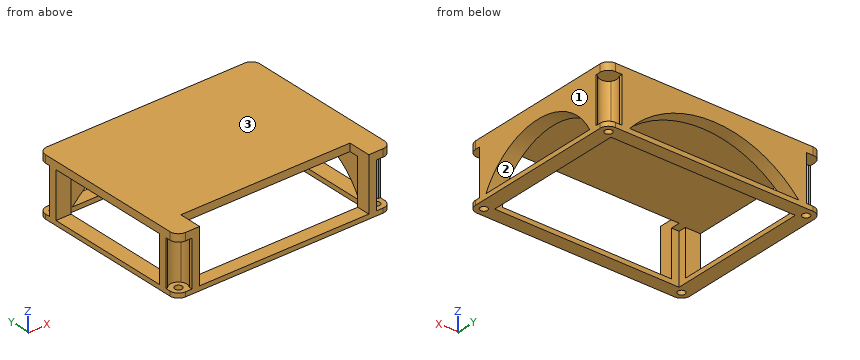
Autodesk Inventor part; units mm, degrees
ref_plane "YZ Plane" through (0, 0, 0) normal (1, 0, 0) x (0, 1, 0)
ref_plane "XZ Plane" through (0, 0, 0) normal (0, 1, 0) x (-1, 0, 0)
ref_plane "XY Plane" through (0, 0, 0) normal (0, 0, 1) x (1, 0, 0)
sketch "Sketch1" plane through (0, 0, 0) normal (0, 0, 1) x (1, 0, 0)
  line L0 (-65, -49.5) -> (65, -49.5) construction
  line L1 (65, -49.5) -> (65, 49.5) construction
  line L2 (65, 49.5) -> (-65, 49.5) construction
  line L3 (-65, 49.5) -> (-65, -49.5) construction
  line L4 (-65, -49.5) -> (65, 49.5) construction
  line L5 (65, -49.5) -> (-65, 49.5) construction
  arc A0 (-65, 55) -> (-70.5, 49.5) centre (-65, 49.5) ccw
  arc A1 (70.5, 49.5) -> (65, 55) centre (65, 49.5) ccw
  arc A2 (65, -55) -> (70.5, -49.5) centre (65, -49.5) ccw
  arc A3 (-70.5, -49.5) -> (-65, -55) centre (-65, -49.5) ccw
  line L6 (-70.5, 49.5) -> (-70.5, -49.5)
  line L7 (-65, -55) -> (65, -55)
  line L8 (70.5, -49.5) -> (70.5, 49.5)
  line L9 (65, 55) -> (-65, 55)
  line L10 (-60.6244, -46.1678) -> (-60.6244, 46.1678)
  line L11 (-60.6244, 46.1678) -> (60.6244, 46.1678)
  line L12 (60.6244, 46.1678) -> (60.6244, -46.1678)
  line L13 (60.6244, -46.1678) -> (-60.6244, -46.1678)
  point P0 (0, 0)
  dimension "d0" = 130
  dimension "d1" = 99
  dimension "d2" = 11
  dimension "d3" = 11
  dimension "d4" = 11
  dimension "d5" = 11
extrude "Extrusion1" add sketch "Sketch1" along normal blind 3
sketch "Sketch2" plane through (0, 0, 3) normal (0, 0, 1) x (1, 0, 0)
  arc A0 (-65, 55) -> (-70.5, 49.5) centre (-65, 49.5) ccw
  circle A1 centre (-65, 49.5) radius 2.4
  arc A2 (70.5, 49.5) -> (65, 55) centre (65, 49.5) ccw
  circle A3 centre (65, 49.5) radius 2.4
  arc A4 (65, -55) -> (70.5, -49.5) centre (65, -49.5) ccw
  circle A5 centre (65, -49.5) radius 2.4
  arc A6 (-70.5, -49.5) -> (-65, -55) centre (-65, -49.5) ccw
  circle A7 centre (-65, -49.5) radius 2.4
  point P0 (0, 0)
  dimension "d8" = 4.8
  dimension "d9" = 4.8
  dimension "d10" = 4.8
  dimension "d11" = 4.8
extrude "Extrusion2" cut sketch "Sketch2" against normal blind 8
sketch "Sketch3" plane through (0, 0, 3) normal (0, 0, 1) x (1, 0, 0)
  circle A0 centre (-65, 49.5) radius 2.4 construction
  circle A1 centre (-65, 49.5) radius 5.5 construction
  circle A2 centre (65, 49.5) radius 2.4 construction
  circle A3 centre (65, 49.5) radius 5.5 construction
  circle A4 centre (65, -49.5) radius 2.4 construction
  circle A5 centre (65, -49.5) radius 5.5 construction
  circle A6 centre (-65, -49.5) radius 2.4 construction
  circle A7 centre (-65, -49.5) radius 5.5 construction
  line L0 (-60.6244, -46.1678) -> (-60.6244, 46.1678)
  line L1 (-65, 55) -> (65, 55)
  line L2 (-60.6244, 52.8322) -> (-60.6244, 55)
  line L3 (-60.6244, 55) -> (60.6244, 55)
  line L4 (60.6244, 55) -> (60.6244, 52.8322)
  line L5 (60.6244, 46.1678) -> (-60.6244, 46.1678)
  arc A8 (-60.6244, 46.1678) -> (-60.6244, 52.8322) centre (-65, 49.5) ccw
  line L6 (60.6244, 46.1678) -> (-60.6244, 46.1678)
  arc A9 (60.6244, 52.8322) -> (60.6244, 46.1678) centre (65, 49.5) ccw
  line L7 (70.5, 49.5) -> (70.5, -49.5)
  line L8 (69.3756, 46.1678) -> (70.5, 46.1678)
  line L9 (70.5, 46.1678) -> (70.5, -46.1678)
  line L10 (70.5, -46.1678) -> (69.3756, -46.1678)
  line L11 (60.6244, -46.1678) -> (60.6244, 46.1678)
  arc A10 (69.3756, -46.1678) -> (60.6244, -46.1678) centre (65, -49.5) ccw
  arc A11 (60.6244, 46.1678) -> (69.3756, 46.1678) centre (65, 49.5) ccw
  line L12 (-70.5, -49.5) -> (-70.5, 49.5)
  line L13 (-69.3756, 46.1678) -> (-70.5, 46.1678)
  line L14 (-70.5, 46.1678) -> (-70.5, 41.1678)
  line L15 (-70.5, 41.1678) -> (-60.6244, 41.1678)
  line L16 (-60.6244, 41.1678) -> (-60.6244, 46.1678)
  arc A12 (-69.3756, 46.1678) -> (-60.6244, 46.1678) centre (-65, 49.5) ccw
  line L17 (-69.3756, -46.1678) -> (-70.5, -46.1678)
  line L18 (-70.5, -46.1678) -> (-70.5, -41.1678)
  line L19 (-70.5, -41.1678) -> (-60.6244, -41.1678)
  line L20 (-60.6244, -41.1678) -> (-60.6244, -46.1678)
  arc A13 (-60.6244, -46.1678) -> (-69.3756, -46.1678) centre (-65, -49.5) ccw
  line L21 (65, -55) -> (-65, -55)
  line L22 (-60.6244, -52.8322) -> (-60.6244, -55)
  line L23 (-60.6244, -55) -> (-55.6244, -55)
  line L24 (-55.6244, -55) -> (-55.6244, -46.1678)
  line L25 (-55.6244, -46.1678) -> (-60.6244, -46.1678)
  line L26 (-60.6244, -46.1678) -> (60.6244, -46.1678)
  arc A14 (-60.6244, -52.8322) -> (-60.6244, -46.1678) centre (-65, -49.5) ccw
  line L27 (60.6244, -52.8322) -> (60.6244, -55)
  line L28 (60.6244, -55) -> (55.6244, -55)
  line L29 (55.6244, -55) -> (55.6244, -46.1678)
  line L30 (55.6244, -46.1678) -> (60.6244, -46.1678)
  arc A15 (60.6244, -46.1678) -> (60.6244, -52.8322) centre (65, -49.5) ccw
  line L31 (-60.6244, 52.8322) -> (-60.6244, 55)
  arc A16 (60.6244, 46.1678) -> (69.3756, 46.1678) centre (65, 49.5) ccw
  line L32 (69.3756, 46.1678) -> (70.5, 46.1678)
  line L33 (70.5, 46.1678) -> (70.5, -46.1678)
  line L34 (70.5, -46.1678) -> (69.3756, -46.1678)
  arc A17 (69.3756, -46.1678) -> (60.6244, -46.1678) centre (65, -49.5) ccw
  line L35 (60.6244, -46.1678) -> (60.6244, 46.1678)
  line L36 (60.6244, -46.1678) -> (60.6244, 46.1678)
  arc A18 (60.6244, 52.8322) -> (60.6244, 46.1678) centre (65, 49.5) ccw
  line L37 (60.6244, 52.8322) -> (60.6244, 55)
  line L38 (60.6244, 55) -> (-60.6244, 55)
  line L39 (-60.6244, 55) -> (-60.6244, 52.8322)
  arc A19 (-60.6244, 46.1678) -> (-60.6244, 52.8322) centre (-65, 49.5) ccw
  line L40 (-60.6244, 46.1678) -> (60.6244, 46.1678)
  line L41 (-60.6244, 46.1678) -> (-60.6244, 41.1678)
  line L42 (-60.6244, 41.1678) -> (-70.5, 41.1678)
  line L43 (-70.5, 41.1678) -> (-70.5, 46.1678)
  line L44 (-70.5, 46.1678) -> (-69.3756, 46.1678)
  arc A20 (-69.3756, 46.1678) -> (-60.6244, 46.1678) centre (-65, 49.5) ccw
  arc A21 (-60.6244, -46.1678) -> (-69.3756, -46.1678) centre (-65, -49.5) ccw
  line L45 (-60.6244, -46.1678) -> (-60.6244, -41.1678)
  line L46 (-60.6244, -41.1678) -> (-70.5, -41.1678)
  line L47 (-70.5, -41.1678) -> (-70.5, -46.1678)
  line L48 (-70.5, -46.1678) -> (-69.3756, -46.1678)
  line L49 (-60.6244, -46.1678) -> (-55.6244, -46.1678)
  line L50 (-55.6244, -46.1678) -> (-55.6244, -55)
  line L51 (-55.6244, -55) -> (-60.6244, -55)
  line L52 (-60.6244, -55) -> (-60.6244, -52.8322)
  arc A22 (-60.6244, -52.8322) -> (-60.6244, -46.1678) centre (-65, -49.5) ccw
  point P0 (0, 0)
  dimension "d14" = 5
  dimension "d15" = 5
  dimension "d16" = 5
  dimension "d17" = 5
extrude "Extrusion3" add sketch "Sketch3" along normal blind 30 contours A13 L17 L12 L19 L0 | L25 L24 L21 L22 A14 | L15 L12 L13 A12 L0 | L26 A15 L27 L21 L29 | A8 L2 L1 L4 A9 L5 | L11 A11 L8 L7 L10 A10
sketch "Sketch4" plane through (-65, 55, 0) normal (0, 1, 0) x (1, 0, 0)
  line L0 (125.6244, -33) -> (4.3756, -33) construction
  line L1 (65, -33) -> (65, -28) construction
  line L2 (124.5, -3) -> (125.6244, -3) construction
  line L3 (125.6244, -3) -> (120.6244, -3) construction
  line L4 (-5.5, -3) -> (4.3756, -3) construction
  line L5 (120.6244, -3) -> (9.3756, -3) construction
  line L6 (4.3756, -3) -> (9.3756, -3) construction
  arc A0 (9.3756, -3) -> (120.6244, -3) centre (65, 46.3814) ccw
  line L7 (9.3756, -3) -> (9.3756, -33)
  line L8 (120.6244, -3) -> (9.3756, -3)
  point P0 (65, 0)
  dimension "d20" = 5
  dimension "d21" = 5
extrude "Extrusion4" cut sketch "Sketch4" against normal blind 10
sketch "Sketch5" plane through (70.5, -49.5, 0) normal (1, 0, 0) x (0, 0, -1)
  line L0 (-33, 95.6678) -> (-33, 3.3322) construction
  line L1 (-33, 49.5) -> (-28, 49.5) construction
  line L2 (0, 3.3322) -> (-3, 3.3322) construction
  line L3 (-3, 8.3322) -> (-3, 90.6678) construction
  line L4 (-3, 3.3322) -> (-3, 8.3322) construction
  line L5 (-3, 95.6678) -> (-33, 95.6678) construction
  line L6 (-3, 95.6678) -> (-3, 90.6678) construction
  line L7 (-3, 90.6678) -> (-33, 90.6678)
  arc A0 (-3, 90.6678) -> (-3, 8.3322) centre (18.3957, 49.5) ccw
  line L8 (-3, 8.3322) -> (-3, 90.6678)
  point P0 (0, 49.5)
  dimension "d24" = 5
extrude "Extrusion5" cut sketch "Sketch5" against normal blind 10
sketch "Sketch6" plane through (0, 0, 33) normal (0, 0, 1) x (1, 0, 0)
  line L0 (70.5, 46.1678) -> (70.5, 49.5) construction
  line L1 (70.5, 46.1678) -> (70.5, 59.6838) construction
  line L2 (-65, -55) -> (65, -55)
  line L3 (70.5, -49.5) -> (70.5, 49.5)
  line L4 (65, 55) -> (-65, 55)
  line L5 (-70.5, 49.5) -> (-70.5, -49.5)
  line L6 (-70.5, -55) -> (70.5, 55) construction
  line L7 (70.5, -55) -> (-70.5, 55) construction
  arc A0 (-65, 55) -> (-70.5, 49.5) centre (-65, 49.5) ccw
  arc A1 (-65, 55) -> (-70.5, 49.5) centre (-65, 49.5) ccw
  line L8 (-70.5, -49.5) -> (-70.5, 49.5)
  arc A2 (-70.5, -49.5) -> (-65, -55) centre (-65, -49.5) ccw
  arc A3 (-70.5, -49.5) -> (-65, -55) centre (-65, -49.5) ccw
  arc A4 (65, -55) -> (70.5, -49.5) centre (65, -49.5) ccw
  arc A5 (65, -55) -> (70.5, -49.5) centre (65, -49.5) ccw
  arc A6 (70.5, 49.5) -> (65, 55) centre (65, 49.5) ccw
  arc A7 (70.5, 49.5) -> (65, 55) centre (65, 49.5) ccw
  point P0 (0, 0)
extrude "Extrusion6" add sketch "Sketch6" along normal blind 5
sketch "Sketch7" plane through (0, 0, 38) normal (0, 0, 1) x (1, 0, 0)
  line L0 (55.6244, -46.1678) -> (55.6244, -55)
  line L1 (55.6244, -55) -> (55.6244, -40)
  line L2 (55.6244, -40) -> (-55.6244, -40)
  line L3 (-55.6244, -40) -> (-55.6244, -55)
  line L4 (-55.6244, -55) -> (55.6244, -55)
  point P0 (0, 0)
  dimension "d29" = 15
extrude "Extrusion7" cut sketch "Sketch7" against normal blind 5
properties part number "CyberDeckHDPower1"
Design review of the part built by this model. Coordinates are the model's own, in mm. Face numbers are marked on the shaded views. Give positions to 0.01 mm unless a question says otherwise; leave off trailing zeros. Loops run counter-clockwise (first coordinate to the right, second up) from the corner with the lowest first, then second, coordinate; pieces in that order, holes last. Notation, with made-up numbers: (-10, -24) -> (40, -24) arc R25 cw to (40, 8) -> close; hole circle Ø1 at (87.25, 82.5). An arc over 180 degrees is marked (long way). One line per item, written item: value.
Q1. For pin 1 Ø2.5 at (y, z) = (54.5, 18) entering from +X; pin 2 Ø4 at (x, y) = (65, -49.5) entering from -Z; pin 3 Ø1.5 at (x, z) = (-19, 30.5) entering from -Y, all flat-tipped, find the tip position at first contact; note any pin that passes through.
Numbers:
pin 1: stops at x = 60.62
pin 2: stops at z = 33
pin 3: stops at y = 46.17
Q2. Draft analysis for pull direction Z (two halves, no side actions). For the marked faces 1, 2 and 3, state which applies: pulls with the +Z half, pulls with the -Z half, needs draft (parallel to the pull), parting line crosses it, or undercut.
Numbers:
face 1: needs draft
face 2: undercut
face 3: pulls with the +Z half
Q3. We need section B-B on x = -49. Give the boundary of the cut face in (y, z).
Numbers:
outline: (-55, 0) -> (-46.17, 0) -> (-46.17, 3) -> (-55, 3) -> close; (-40, 33) -> (46.17, 33) -> (46.17, 9.58) -> (55, 9.58) -> (55, 38) -> (-40, 38) -> close; (46.17, 0) -> (55, 0) -> (55, 3) -> (46.17, 3) -> close
Q4. We need section A-A on y = -28.5. Give the boundary of the cut face in (x, z).
Numbers:
outline: (-70.5, 0) -> (-60.62, 0) -> (-60.62, 3) -> (-70.5, 3) -> close; (-70.5, 33) -> (60.62, 33) -> (60.62, 18.21) -> (70.5, 18.21) -> (70.5, 38) -> (-70.5, 38) -> close; (60.62, 0) -> (70.5, 0) -> (70.5, 3) -> (60.62, 3) -> close
Q5. For L1, parallel to Y at x = -65, z = 1.05; L2, parallel to Z at x = 62.5, y = -1.5; L3, parallel to Y at x = -63.5, z = 2, list the stretches that pass through material, from the lowest coordinate up.
Numbers:
L1: y = -55 to -51.9, -47.1 to 47.1, 51.9 to 55
L2: z = 0 to 3, 27.98 to 38
L3: y = -55 to -51.37, -47.63 to 47.63, 51.37 to 55
